Geometry: see drawing. Coordinates: mm, zero at the bounding-box minimum. A direction names the side the tool comes from. Coordinates: 2 decimals unless noted, no trailing zeros. Write each loop counter-clockwise with the first axis right and the second up, starting at its lowest first coordinate (ties: lowest second). Pieces come first, ordered by that corner, then holes.
1) Section query A-A (y = 142). Output: boundary loops of the cut face in (x, z).
2) Draft query along X for the marked faces 5, 6 and 7. Return one class per face: pulls with the +X half, pulls with the -X half, needs draft (parallel to the pull), parting line crosses it, or undercut.
3) Section query D-D (y = 761.5). Output: boundary loops of the cut face in (x, z).
4) Section query B-B (x = 884). Output: boundary loops of the cut face in (y, z), then the cut area to 3 significant figures.
5) Pin query (flat end, axial travel): pin 1 Ø3 at (x, y) = (562, 742.5) entering from +Z; pin 2 Ø10 at (y, z) = (321, 81) entering from +X; pin 3 Ø6 at (y, z) = (436, 137) entering from -X; pin 4 Ø3 at (x, z) = (342.5, 64) entering from -Y. Return the tip coordinate at first contact, or that it passes through.
6) Line query: L1, parallel to Z at x = 375.5, y = 358; L2, parallel to X at y = 185.5, z = 107; L3, parallel to Y at x = 858, z = 35. Output: solid intervals per line, ascending.
7) Section query C-C (z = 17). Output: boundary loops of the cut face in (x, y), then the cut area to 3 significant figures.
8) Set-up query: the marked faces 1, 2, 3 and 4. Return all of +Z, -Z, +X, -X, +Y, -Y with unobstructed straight access to the full face (end or side cutting, diameter ignored); none if empty.
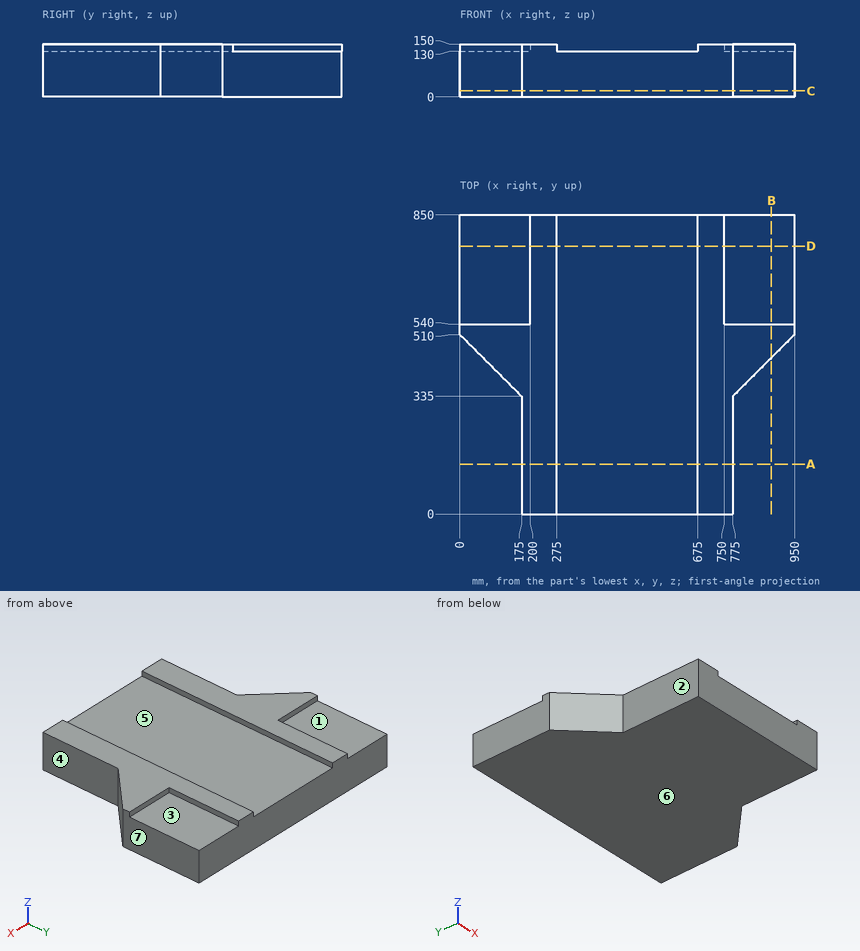
Answer:
1. outline: (175, 0) - (775, 0) - (775, 150) - (675, 150) - (675, 130) - (275, 130) - (275, 150) - (175, 150) - close
2. face 5: undercut
2. face 6: needs draft
2. face 7: pulls with the +X half
3. outline: (0, 0) - (950, 0) - (950, 130) - (750, 130) - (750, 150) - (675, 150) - (675, 130) - (275, 130) - (275, 150) - (200, 150) - (200, 130) - (0, 130) - close
4. outline: (444, 0) - (850, 0) - (850, 130) - (540, 130) - (540, 150) - (444, 150) - close
4. area: 54,700 mm2
5. pin 1: stops at z = 130
5. pin 2: stops at x = 775
5. pin 3: stops at x = 71
5. pin 4: stops at y = 0
6. L1: z = 0 to 130
6. L2: x = 175 to 775
6. L3: y = 418 to 850
7. outline: (0, 510) - (175, 335) - (175, 0) - (775, 0) - (775, 335) - (950, 510) - (950, 850) - (0, 850) - close
7. area: 660,000 mm2
8. face 1: +Z, -X, +Y
8. face 2: +Z, -Z, -X, -Y
8. face 3: +Z, +X, +Y
8. face 4: +Z, -Z, +X, -Y
